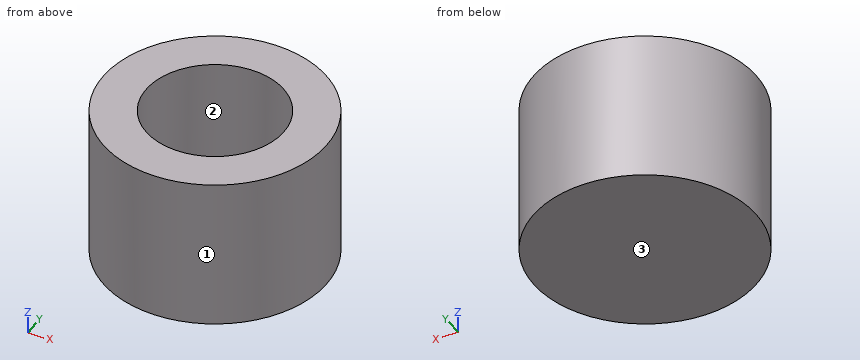
from build123d import *

# Parameters (mm, degrees)
SKETCH1_R           = 20.2565
SKETCH1_R_2         = 12.499975
BOSS_EXTRUDE1_DEPTH = 27.686
SHELL1_T            = -0.254
SKETCH2_R           = 12.499975
BOSS_EXTRUDE2_DEPTH = 0.254
BOSS_EXTRUDE3_START = -0.254
SKETCH3_R           = 20.0025
SKETCH3_R_2         = 12.753975
BOSS_EXTRUDE3_DEPTH = 0.254


with BuildPart() as part:
    # Sketch1 → Boss-Extrude1 (new body)
    with BuildSketch(Plane.XY):
        Circle(SKETCH1_R)
        Circle(SKETCH1_R_2, mode=Mode.SUBTRACT)
    extrude(amount=BOSS_EXTRUDE1_DEPTH)

    # Shell1
    shell1_openings = [part.faces().sort_by_distance(p)[0] for p in [
        (-19.683559659, 0, 27.686),
    ]]
    offset(amount=SHELL1_T, openings=shell1_openings, kind=Kind.INTERSECTION)

    # Sketch2 → Boss-Extrude2 (add)
    with BuildSketch(Plane(origin=(0, 0, 0), x_dir=(-1, 0, 0), z_dir=(0, 0, -1))):
        Circle(SKETCH2_R)
    extrude(amount=-BOSS_EXTRUDE2_DEPTH)

    # Sketch3 → Boss-Extrude3 (add)
    with BuildSketch(Plane.XY.offset(27.686).offset(BOSS_EXTRUDE3_START)):
        Circle(SKETCH3_R)
        Circle(SKETCH3_R_2, mode=Mode.SUBTRACT)
    extrude(amount=BOSS_EXTRUDE3_DEPTH)


solid = part.part
Could you check a few things on this model? Use its own coordinates, in mm. Face numbers are marked on the shaded views. Coordinates: 2 decimals unless noted, no trailing zeros. Write each loop counter-clockwise with the first axis right and the second up, starting at its lowest first coordinate (ties: lowest second). Pieces come first, ordered by that corner, then holes. Notation, with made-up numbers: (-9, 33.25) - (38, 33.25) arc R22 cw to (38, 49.25) - close; hole circle Ø7 at (49.5, 86.5). An arc over 180 degrees is marked (long way). Put each result on its own line as item: value. Start each with the question number.
Q1. I want a section at A-A on z = 6.5. Write out the boundary of the cut face in (x, y) (1 decimal), plus the area to 3 significant figures.
Q2. I'm going to push flat-ended pins straight in: P1, Ø6, axis at x = -3.5, z = 22.5, coming from the +Y side; P2, Ø1, axis at y = 2, z = 8, coming from the -X side; P3, Ø15, axis at x = 0, y = 0, coming from the +Z side; P4, Ø5, axis at x = -3.5, y = 16, coming from the -Z side. Where does each tip first touch, or does it pass through?
Q3. Thinking about a two-plate mould opening in Y: for the marked faces 1, 2 and 3, which applies, pulls with the +Y half, pulls with the -Y half, needs draft (parallel to the pull), parting line crosses it, or undercut?
Q4. I want a section at B-B on x = 0. Write out the boundary of the cut face in (y, z).
Q5. I want a section at D-D on y = 14.5. Write out the boundary of the cut face in (x, z).
Q6. Please list where these lines run through material, in increasing order: L1, parallel to Y at x = 0, z = 17.5; L2, parallel to Z at x = -8.5, y = -18; L3, parallel to X at y = 3, z = 18.5.
Checks:
1. outline: circle Ø40.5 at (0, 0); circle Ø25.5 at (0, 0); hole circle Ø40 at (0, 0); hole circle Ø25 at (0, 0)
1. area: 52.3 mm²
2. P1: y = 20.25
2. P2: x = -20.2
2. P3: z = 0.25
2. P4: z = 0
3. face 1: parting line crosses it
3. face 2: undercut
3. face 3: needs draft
4. outline: (-20.26, 0) - (20.26, 0) - (20.26, 27.69) - (12.5, 27.69) - (12.5, 0.25) - (-12.5, 0.25) - (-12.5, 27.69) - (-20.26, 27.69) - close; hole (-20, 0.25) - (-12.75, 0.25) - (-12.75, 27.43) - (-20, 27.43) - close; hole (12.75, 0.25) - (20, 0.25) - (20, 27.43) - (12.75, 27.43) - close
5. outline: (-14.14, 0) - (14.14, 0) - (14.14, 27.69) - (-14.14, 27.69) - close; hole (-13.78, 0.25) - (13.78, 0.25) - (13.78, 27.43) - (-13.78, 27.43) - close
6. L1: -20.26 to -20, -12.75 to -12.5, 12.5 to 12.75, 20 to 20.26
6. L2: 0 to 0.25, 27.43 to 27.69
6. L3: -20.03 to -19.78, -12.4 to -12.13, 12.13 to 12.4, 19.78 to 20.03
